from build123d import *

# Parameters (mm, degrees)
F1_DEPTH    = 25.4
F2_T1_DEPTH = 76.2


# Not quite as in the source:
# - a fillet or chamfer that OpenCascade refuses, or shapes differently, is made with other operations: its cross-section is extruded or revolved along the edge and cut away or added


with BuildPart() as f1:
    # F0 (on Front) → F1 (new body)
    with BuildSketch(Plane.XZ):
        with BuildLine():
            Line((-12.7, 25.4), (-25.4, 25.4))
            Line((-25.4, 25.4), (-25.4, 12.798297219))
            Line((-25.4, 12.798297219), (-21.59, 12.798297219))
            ThreePointArc((-21.59, 12.798297219), (-18.9861792847, 19.0844765037), (-12.7, 21.688297219))
            Line((-12.7, 21.688297219), (-12.7, 25.4))
        make_face()
        with BuildLine():
            Line((0, 25.4), (-12.7, 25.4))
            Line((-12.7, 25.4), (-12.7, 21.688297219))
            ThreePointArc((-12.7, 21.688297219), (-6.4138207153, 19.0844765037), (-3.81, 12.798297219))
            Line((-3.81, 12.798297219), (0, 12.798297219))
            Line((0, 12.798297219), (0, 25.4))
        make_face()
        with BuildLine():
            Line((-21.59, 12.798297219), (-25.4, 12.798297219))
            Line((-25.4, 12.798297219), (-25.4, 0))
            Line((-25.4, 0), (-12.7, 0))
            Line((-12.7, 0), (-12.7, 3.908297219))
            ThreePointArc((-12.7, 3.908297219), (-18.9861792847, 6.5121179342), (-21.59, 12.798297219))
        make_face()
        with BuildLine():
            Line((12.5505886972, 25.4), (0, 25.4))
            Line((0, 25.4), (0, 12.798297219))
            Line((0, 12.798297219), (3.6976524143, 12.798297219))
            ThreePointArc((3.6976524143, 12.798297219), (6.2922356041, 19.0752253837), (12.5615055494, 21.6882587679))
            Line((12.5615055494, 21.6882587679), (12.5505886972, 25.4))
        make_face()
        with BuildLine():
            Line((-12.7, 0), (-25.4, 0))
            Line((-25.4, 0), (-25.4, -12.798297219))
            Line((-25.4, -12.798297219), (-21.59, -12.798297219))
            ThreePointArc((-21.59, -12.798297219), (-18.9861792847, -6.5121179342), (-12.7, -3.908297219))
            Line((-12.7, -3.908297219), (-12.7, 0))
        make_face()
        with BuildLine():
            Line((25.4, 25.4), (12.5505886972, 25.4))
            Line((12.5505886972, 25.4), (12.5615055494, 21.6882587679))
            ThreePointArc((12.5615055494, 21.6882587679), (18.8645805791, 19.0937140292), (21.4776524143, 12.798297219))
            Line((21.4776524143, 12.798297219), (25.4, 12.798297219))
            Line((25.4, 12.798297219), (25.4, 25.4))
        make_face()
        with BuildLine():
            Line((-21.59, -12.798297219), (-25.4, -12.798297219))
            Line((-25.4, -12.798297219), (-25.4, -25.4))
            Line((-25.4, -25.4), (-12.7, -25.4))
            Line((-12.7, -25.4), (-12.7, -21.688297219))
            ThreePointArc((-12.7, -21.688297219), (-18.9861792847, -19.0844765037), (-21.59, -12.798297219))
        make_face()
        with BuildLine():
            Line((25.4, 0), (25.4, 12.798297219))
            Line((25.4, 12.798297219), (21.4776524143, 12.798297219))
            ThreePointArc((21.4776524143, 12.798297219), (18.8830692245, 6.5213690542), (12.6137992792, 3.90833567))
            Line((12.6137992792, 3.90833567), (12.6252943486, 0))
            Line((12.6252943486, 0), (25.4, 0))
        make_face()
        with BuildLine():
            Line((3.7729362829, -12.798297219), (0, -12.798297219))
            Line((0, -12.798297219), (0, -25.4))
            Line((0, -25.4), (12.7, -25.4))
            Line((12.7, -25.4), (12.6890831478, -21.6882587679))
            ThreePointArc((12.6890831478, -21.6882587679), (6.3860081181, -19.0937140292), (3.7729362829, -12.798297219))
        make_face()
        with BuildLine():
            Line((0, -25.4), (0, -12.798297219))
            Line((0, -12.798297219), (-3.81, -12.798297219))
            ThreePointArc((-3.81, -12.798297219), (-6.4138207153, -19.0844765037), (-12.7, -21.688297219))
            Line((-12.7, -21.688297219), (-12.7, -25.4))
            Line((-12.7, -25.4), (0, -25.4))
        make_face()
        with BuildLine():
            Line((25.4, 0), (12.6252943486, 0))
            Line((12.6252943486, 0), (12.636789418, -3.90833567))
            ThreePointArc((12.636789418, -3.90833567), (18.9398644476, -6.5028804088), (21.5529362829, -12.798297219))
            Line((21.5529362829, -12.798297219), (25.4, -12.798297219))
            Line((25.4, -12.798297219), (25.4, 0))
        make_face()
        with BuildLine():
            Line((25.4, -25.4), (25.4, -12.798297219))
            Line((25.4, -12.798297219), (21.5529362829, -12.798297219))
            ThreePointArc((21.5529362829, -12.798297219), (18.9583530931, -19.0752253837), (12.6890831478, -21.6882587679))
            Line((12.6890831478, -21.6882587679), (12.7, -25.4))
            Line((12.7, -25.4), (25.4, -25.4))
        make_face()
        with BuildLine():
            Line((3.6976524143, 12.798297219), (0, 12.798297219))
            Line((0, 12.798297219), (0, 0))
            Line((0, 0), (12.6252943486, 0))
            Line((12.6252943486, 0), (12.6137992792, 3.90833567))
            ThreePointArc((12.6137992792, 3.90833567), (6.3107242496, 6.5028804088), (3.6976524143, 12.798297219))
        make_face()
        with BuildLine():
            Line((12.6252943486, 0), (0, 0))
            Line((0, 0), (0, -12.798297219))
            Line((0, -12.798297219), (3.7729362829, -12.798297219))
            ThreePointArc((3.7729362829, -12.798297219), (6.3675194726, -6.5213690542), (12.636789418, -3.90833567))
            Line((12.636789418, -3.90833567), (12.6252943486, 0))
        make_face()
        with BuildLine():
            Line((0, 0), (0, 12.798297219))
            Line((0, 12.798297219), (-3.81, 12.798297219))
            ThreePointArc((-3.81, 12.798297219), (-6.4138207153, 6.5121179342), (-12.7, 3.908297219))
            Line((-12.7, 3.908297219), (-12.7, 0))
            Line((-12.7, 0), (0, 0))
        make_face()
        with BuildLine():
            Line((0, 0), (-12.7, 0))
            Line((-12.7, 0), (-12.7, -3.908297219))
            ThreePointArc((-12.7, -3.908297219), (-6.4138207153, -6.5121179342), (-3.81, -12.798297219))
            Line((-3.81, -12.798297219), (0, -12.798297219))
            Line((0, -12.798297219), (0, 0))
        make_face()
    extrude(amount=F1_DEPTH)

    # F2: fillet of radius 5.08 on 1 edges, made by hand

    # F2_s2 → F2_t1 (cut)
    with BuildSketch(Plane.YZ.offset(-38.1)):
        with BuildLine():
            ThreePointArc((-20.32, 25.4), (-23.9121024484, 23.9121024484), (-25.4, 20.32))
            Line((-25.4, 20.32), (-25.4, 25.4))
            Line((-25.4, 25.4), (-20.32, 25.4))
        make_face()
    extrude(amount=F2_T1_DEPTH, mode=Mode.SUBTRACT)


solid = f1.part
Model file for the job. Use its own axes, mm. Round coordinates to 2 decimals unless told otherwise and drop trailing zeros. Order: outer loops, then holes, each group sorted by start corner. A loop starts at its lowest first (then second) coordinate and runs counter-clockwise, first axis right, second up.
(1) Band-saw the part on D-D (y = -23.75). List the corners of the cut face in (x, z), then the cut area to 3 significant figures.
(2) Band-saw the part on B-B (y = -10.25). List the corners of the cut face in (x, z).
(3) Band-saw the part on A-A (z = 7). List the corners of the cut face in (x, y).
(4) Drill centre lines: line 1 (Z direction, x = -15, y = -16.5); line 2 (Z direction, x = 20.5, y = -9); line 3 (X direction, y = -15.5, z = 14.5). Where is each one in solid material? Low to high.
(5) Band-saw the part on C-C (x = 9). List the corners of the cut face in (y, z).
Verdict:
1. outline: (-25.4, -25.4) - (25.4, -25.4) - (25.4, 24.07) - (-25.4, 24.07) - close; hole circle Ø17.78 at (-12.7, -12.8); hole circle Ø17.78 at (-12.7, 12.8); hole circle Ø17.78 at (12.59, 12.8); hole circle Ø17.78 at (12.66, -12.8)
1. area: 1,520 mm2
2. outline: (-25.4, -25.4) - (25.4, -25.4) - (25.4, 25.4) - (-25.4, 25.4) - close; hole circle Ø17.78 at (-12.7, -12.8); hole circle Ø17.78 at (-12.7, 12.8); hole circle Ø17.78 at (12.59, 12.8); hole circle Ø17.78 at (12.66, -12.8)
3. outline: (-25.4, -25.4) - (-19.44, -25.4) - (-19.44, 0) - (-25.4, 0) - close; (-5.96, -25.4) - (5.85, -25.4) - (5.85, 0) - (-5.96, 0) - close; (19.33, -25.4) - (25.4, -25.4) - (25.4, 0) - (19.33, 0) - close
4. line 1: z = -25.4 to -21.39, -4.21 to 4.21, 21.39 to 25.4
4. line 2: z = -25.4 to -17, -8.6 to 8.75, 16.85 to 25.4
4. line 3: x = -25.4 to -21.43, -3.97 to 3.86, 21.31 to 25.4
5. outline: (-25.4, -25.4) - (0, -25.4) - (0, -20.9) - (-25.4, -20.9) - close; (-25.4, -4.7) - (0, -4.7) - (0, 4.66) - (-25.4, 4.66) - close; (-25.36, 20.93) - (0, 20.93) - (0, 25.4) - (-20.32, 25.4) arc R5.08 ccw to start
